```python
from build123d import *

# Parameters (mm, degrees)
SKETCH1_W           = 40
SKETCH1_H           = 40
BOSS_EXTRUDE1_DEPTH = 500
SKETCH2_R           = 3
FILLET1_R           = 5
SKETCH4_W           = 26.319455472
SKETCH4_H           = 27.036606846
CUT_EXTRUDE1_DEPTH  = 484
SKETCH5_W           = 49.254498594
SKETCH5_H           = 49.142556558
BOSS_EXTRUDE3_DEPTH = 11
SKETCH6_R           = 8
CUT_EXTRUDE2_DEPTH  = 149


with BuildPart() as part:
    # Sketch1 → Boss-Extrude1 (new body)
    with BuildSketch(Plane.XY):
        Rectangle(SKETCH1_W, SKETCH1_H)
    extrude(amount=BOSS_EXTRUDE1_DEPTH)

    # Sketch2 → Revolve1 (revolve)
    with BuildSketch(Plane.XY.offset(500), mode=Mode.PRIVATE) as revolve1_sk:
        with Locations((-10, 0)):
            Circle(SKETCH2_R)
    revolve(revolve1_sk.sketch.rotate(Axis((0, 23.495779736, 500), (0, -1, 0)), 270), axis=Axis((0, 23.495779736, 500), (0, -1, 0)))

    # Fillet1
    fillet1_edges = [part.edges().sort_by_distance(p)[0] for p in [
        (20, -20, 250),
        (-20, -20, 250),
        (-20, 20, 250),
        (20, 20, 250),
    ]]
    fillet(fillet1_edges, radius=FILLET1_R)

    # Sketch4 → Cut-Extrude1 (cut)
    with BuildSketch(Plane(origin=(0, 0, 0), x_dir=(-1, 0, 0), z_dir=(0, 0, -1))):
        Rectangle(SKETCH4_W, SKETCH4_H)
    extrude(amount=-CUT_EXTRUDE1_DEPTH, mode=Mode.SUBTRACT)

    # Sketch5 → Boss-Extrude3 (add)
    with BuildSketch(Plane(origin=(0, 0, 0), x_dir=(-1, 0, 0), z_dir=(0, 0, -1))):
        Rectangle(SKETCH5_W, SKETCH5_H)
    extrude(amount=BOSS_EXTRUDE3_DEPTH)

    # Sketch6 → Cut-Extrude2 (cut)
    with BuildSketch(Plane(origin=(20, 0, 0), x_dir=(0, 0, -1), z_dir=(1, 0, 0))):
        with Locations((-65.399193922, 0)):
            Circle(SKETCH6_R)
        with Locations((-304.968679319, 0)):
            Circle(SKETCH6_R)
        with Locations((-334.968679319, 0)):
            Circle(SKETCH6_R)
        with Locations((-364.968679319, 0)):
            Circle(SKETCH6_R)
        with Locations((-394.968679319, 0)):
            Circle(SKETCH6_R)
        with Locations((-424.968679319, 0)):
            Circle(SKETCH6_R)
    extrude(amount=-CUT_EXTRUDE2_DEPTH, mode=Mode.SUBTRACT)


solid = part.part
```
For this review, take the finished solid that the model builds, in its own axes (mm). A direction names the side the tool comes from. Give positions to 0.01 mm unless a question says otherwise; leave off trailing zeros. Write each loop counter-clockwise with the first axis right and the second up, starting at its lowest first coordinate (ties: lowest second). Pieces come first, ordered by that corner, then holes.
Item 1: The part is to be moulded in two halves that separate along Z. For faces 5 (the face through (0, 24.571, -5)), 6 (the face through (0, -21, 0)), 7 (the face through (16.63, 0.35, 342.96)), say which applies: +Z half, -Z half, draft (parallel to the pull), parting line (faces both ways), or undercut.
Item 2: Insertion check: P1, Ø21.5, axis at y = 3, z = 154, coming from the +X side; P2, Ø3, axis at x = 6.5, z = 234, coming from the -Y side; P3, Ø18.5, axis at y = 0, z = 334.97, coming from the -X side; P4, Ø21, axis at x = 0, y = 6, coming from the +Z side. Each pin has a flat end and moves straight along its axis. Give the tip position at first contact, or say it passes through.
Item 3: Take a section at C-C (z = 69). Give the boundary of the cut face in (x, y), and give its area (3 significant figures).
Item 4: Wall thickness on probe 1 along Z at (x, y) = (3, 6.5); probe 2 along Y at (x, z) = (-9, 166.5); probe 3 along X at (y, z) = (0, 483): over which ranges is each line inside the solid? List them lowest first.
Item 5: Take a section at A-A (z = 422.5). Give the boundary of the cut face in (x, y), and give its area (3 significant figures).
Item 6: Machinability: for faces 1 (the face through (20, 0, 246)), 2 (the face through (-16.53, 0.35, 342.96)), 3 (the face through (0, -20, 246)), 4 (the face through (0, 13.518, 239)), which of the approach directions +Z, -Z, +X, -X, +Y, -Y give a long, thin tool a straight path to every point of the face, cutting with its end or side? Answer none if there is none.
Item 7: Take a section at B-B (z = 134.5). Give the boundary of the cut face in (x, y), and give its area (3 significant figures).
Established:
1. face 5: draft
1. face 6: +Z half
1. face 7: undercut
2. P1: stops at x = 20
2. P2: stops at y = -20
2. P3: stops at x = -20
2. P4: stops at z = 513
3. outline: (-20, -15) arc R5 ccw to (-15, -20) - (15, -20) arc R5 ccw to (20, -15) - (20, -7.14) - (13.16, -7.14) - (13.16, -13.52) - (-13.16, -13.52) - (-13.16, -7.14) - (-20, -7.14) - close; (-20, 7.14) - (-13.16, 7.14) - (-13.16, 13.52) - (13.16, 13.52) - (13.16, 7.14) - (20, 7.14) - (20, 15) arc R5 ccw to (15, 20) - (-15, 20) arc R5 ccw to (-20, 15) - close
3. area: 671 mm2
4. probe 1: z = -11 to 0, 484 to 500
4. probe 2: y = -20 to -13.52, 13.52 to 20
4. probe 3: x = -20 to -13.16, 13.16 to 20
5. outline: (-20, -15) arc R5 ccw to (-15, -20) - (15, -20) arc R5 ccw to (20, -15) - (20, -7.61) - (13.16, -7.61) - (13.16, -13.52) - (-13.16, -13.52) - (-13.16, -7.61) - (-20, -7.61) - close; (-20, 7.61) - (-13.16, 7.61) - (-13.16, 13.52) - (13.16, 13.52) - (13.16, 7.61) - (20, 7.61) - (20, 15) arc R5 ccw to (15, 20) - (-15, 20) arc R5 ccw to (-20, 15) - close
5. area: 659 mm2
6. face 1: +Z, +X, +Y, -Y
6. face 2: +X, -X
6. face 3: +Z, +X, -X, -Y
6. face 4: none
7. outline: (-20, -15) arc R5 ccw to (-15, -20) - (15, -20) arc R5 ccw to (20, -15) - (20, 15) arc R5 ccw to (15, 20) - (-15, 20) arc R5 ccw to (-20, 15) - close; hole (-13.16, -13.52) - (13.16, -13.52) - (13.16, 13.52) - (-13.16, 13.52) - close
7. area: 867 mm2
